Geometry: final body of the model. Coordinates: model frame, mm. Coordinates: 2 decimals unless noted, no trailing zeros. Loops run counter-clockwise (first coordinate to the right, second up) from the corner with the lowest first, then second, coordinate; pieces in that order, holes last. Notation, with made-up numbers: (9.5, -8.5) - (48.5, -8.5) arc R27 ccw to (48.5, 24.5) - close; hole circle Ø7 at (-34.5, 60). An arc over 180 degrees is marked (long way). Return JSON: item names as keys, results as strings.
Autodesk Inventor part; units mm, degrees
ref_plane "YZ Plane" through (0, 0, 0) normal (1, 0, 0) x (0, 1, 0)
ref_plane "XZ Plane" through (0, 0, 0) normal (0, 1, 0) x (-1, 0, 0)
ref_plane "XY Plane" through (0, 0, 0) normal (0, 0, 1) x (1, 0, 0)
sketch "Sketch1" plane through (0, 0, 0) normal (0, 0, 1) x (1, 0, 0)
  line L0 (0, 0) -> (25.5, 0)
  line L1 (25.5, 0) -> (25.5, 10)
  line L2 (25.5, 10) -> (21, 10)
  line L3 (21, 10) -> (20, 9)
  line L4 (20, 9) -> (3, 9)
  line L5 (3, 9) -> (2, 10)
  line L6 (2, 10) -> (0, 10)
  line L7 (0, 10) -> (0, 0)
  dimension "d0" = 25.5
  dimension "d1" = 9
  dimension "d2" = 17
  dimension "d3" = 1
  dimension "d4" = 2
revolve "Revolution1" add sketch "Sketch1" angle 360 about axis through (0, 0, 0) along (1, 0, 0)
sketch "Sketch2" plane through (25.5, 0, 0) normal (1, 0, 0) x (0, 0, -1)
  circle A0 centre (0, 0) radius 10
  circle A1 centre (0, 0) radius 2.5
  dimension "d6" = 5
extrude "Extrusion1" cut sketch "Sketch2" against normal through all contours A1
properties part number "spool"
Item 1: Ray query, probe 1 along Y at (x, z) = (16.25, 2); probe 2 along X at (y, z) = (-6, -7.75); probe 3 along Z at (x, y) = (14.75, -1.5). Return the intervals inside material, ascending. Write a range as from..to.
Worked out:
{"probe 1": "-8.77..-1.5, 1.5..8.77", "probe 2": "0..2.2, 20.8..25.5", "probe 3": "-8.87..-2, 2..8.87"}
Item 2: Mould query, pull axis X, two halves, no side actions, for faces 1 (the face through (11.381, -1.172, -8.923)), 2 (the face through (23.22, -2.17, 9.76)), 3 (the face through (0, 2, -2)). Classes: +X half, -X half, draft (parallel to the pull), parting line (faces both ways), or undercut.
Worked out:
{"face 1": "undercut", "face 2": "draft", "face 3": "-X half"}
Item 3: First-contact query: pin 1 Ø4 at (x, y) = (21.5, -3) entering from +Z; pin 2 Ø2 at (x, y) = (9, 7.5) entering from +Z; pin 3 Ø2 at (x, y) = (13.5, 1.5) entering from -Z; pin 4 Ø12 at (x, z) = (19, -5) entering from -Y. Flat tips, straight axial feed; report the tip coordinate or a pass-through.
Worked out:
{"pin 1": "z = 9.95", "pin 2": "z = 6.22", "pin 3": "z = -8.99", "pin 4": "y = -10"}
Item 4: Section query D-D, the plane x = 21.5. Return loops of the section in (y, z).
Worked out:
{"outline": "circle Ø20 at (0, 0); hole circle Ø5 at (0, 0)"}
Item 5: Section query A-A, the plane y = 0. Return loops of the section in (x, z), and give its area (4 significant figures).
Worked out:
{"outline": "(0, -10) - (2, -10) - (3, -9) - (20, -9) - (21, -10) - (25.5, -10) - (25.5, -2.5) - (0, -2.5) - close; (0, 2.5) - (25.5, 2.5) - (25.5, 10) - (21, 10) - (20, 9) - (3, 9) - (2, 10) - (0, 10) - close", "area": "346.5 mm^2"}
Item 6: Section query C-C, the plane x = 5.25. Return loops of the section in (y, z).
Worked out:
{"outline": "circle Ø18 at (0, 0); hole circle Ø5 at (0, 0)"}
